Autodesk Inventor part; units mm, degrees
ref_plane "YZ Plane" through (0, 0, 0) normal (1, 0, 0) x (0, 1, 0)
ref_plane "XZ Plane" through (0, 0, 0) normal (0, 1, 0) x (-1, 0, 0)
ref_plane "XY Plane" through (0, 0, 0) normal (0, 0, 1) x (1, 0, 0)
ref_plane "Work Plane1" through (-1.5, 0, 1210) normal (-1, 0, 0) x (0, 0, 1)
sketch "Sketch1" plane through (-1.5, 0, 1210) normal (-1, 0, 0) x (0, 0, 1)
  circle A0 centre (-606.5, 339) radius 1.5
  circle A1 centre (-848.5, 64) radius 1.5
  circle A2 centre (-1090.5, 339) radius 1.5
  circle A3 centre (-848.5, 614) radius 1.5
  circle A4 centre (-364.5, 614) radius 1.5
  circle A5 centre (-364.5, 64) radius 1.5
  circle A6 centre (-122.5, 339) radius 1.5
  circle A7 centre (-122.5, 614) radius 1.5
  circle A8 centre (-122.5, 64) radius 1.5
  circle A9 centre (-364.5, 339) radius 1.5
  circle A10 centre (-606.5, 614) radius 1.5
  circle A11 centre (-1090.5, 614) radius 1.5
  circle A12 centre (-1090.5, 64) radius 1.5
  circle A13 centre (-848.5, 339) radius 1.5
  circle A14 centre (-606.5, 64) radius 1.5
  line L0 (-1211.5, 0) -> (0, 0)
  line L1 (0, 0) -> (0, 1000)
  line L2 (-1211.5, 1000) -> (0, 1000)
  line L3 (-1211.5, 0) -> (-1211.5, 1000)
  line L4 (-25, 76.5) -> (-1186.5, 76.5)
  line L5 (-1186.5, 76.5) -> (-1186.5, 51.5)
  line L6 (-1186.5, 51.5) -> (-25, 51.5)
  line L7 (-25, 51.5) -> (-25, 76.5)
  line L8 (-122.5, 64) -> (-114.6022, 64)
  point P0 (-1210, 0)
  dimension "d0" = 25
  dimension "d1" = 25
  dimension "d2" = 25
ref_plane "Work Plane2" through (-1211.5, 0, -1.5) normal (1, 0, 0) x (0, 0, -1)
sketch "Sketch2" plane through (-1211.5, 0, -1.5) normal (1, 0, 0) x (0, 0, -1)
  line L0 (-25, 51.5) -> (-1186.5, 51.5)
  line L1 (-25, 76.5) -> (-25, 51.5)
  line L2 (-1186.5, 76.5) -> (-25, 76.5)
  line L3 (-1186.5, 51.5) -> (-1186.5, 76.5)
  circle A0 centre (-121, 64) radius 1.5
  circle A1 centre (-363, 64) radius 1.5
  circle A2 centre (-605, 64) radius 1.5
  circle A3 centre (-847, 64) radius 1.5
  circle A4 centre (-1089, 64) radius 1.5
  point P0 (-1.5, 0)
extrude "Extrusion1" add sketch "Sketch2" along normal blind 25
extrude "Extrusion2" add sketch "Sketch1" along normal blind 25 contours L7 L6 L5 L4
ref_plane "Work Plane3" through (-1.5, 0, 1210) normal (-1, 0, 0) x (0, 0, 1)
sketch "Sketch3" plane through (-1.5, 0, 1210) normal (-1, 0, 0) x (0, 0, 1)
  line L0 (-1186.5, 76.5) -> (-1186.5, 51.5)
  line L1 (-1186.5, 51.5) -> (-1210, 51.5)
  line L2 (-1210, 51.5) -> (-1210, 76.5)
  line L3 (-1210, 76.5) -> (-1186.5, 76.5)
  line L4 (-1186.5, 76.5) -> (-1186.5, 51.5)
  line L5 (-1.5, 0) -> (-1.5, 1000)
  line L6 (-25, 76.5) -> (-25, 51.5)
  line L7 (-25, 51.5) -> (-1.5, 51.5)
  line L8 (-1.5, 51.5) -> (-1.5, 76.5)
  line L9 (-1.5, 76.5) -> (-25, 76.5)
  line L10 (-25, 76.5) -> (-25, 51.5)
  point P0 (-1210, 0)
extrude "Extrusion3" add sketch "Sketch3" along normal up to surface (1210 mm away)
sketch "Sketch4" plane through (-1.5, 51.5, 1208.5) normal (0, 0, 1) x (1, 0, 0)
  circle A0 centre (-121, 12.5) radius 1.5
  circle A1 centre (-363, 12.5) radius 1.5
  circle A2 centre (-605, 12.5) radius 1.5
  circle A3 centre (-847, 12.5) radius 1.5
  circle A4 centre (-1089, 12.5) radius 1.5
  point P0 (1.5, -51.5)
hole "Hole1" at (-122.5, 64, 1208.5) at (-606.5, 64, 1208.5) at (-364.5, 64, 1208.5) at (-848.5, 64, 1208.5) at (-1090.5, 64, 1208.5) direction (0, 0, -1) diameter 3 end through all
properties part number "HoneyComb Frame"
For this review, take the finished solid that the model builds, in its own axes (mm). Round coordinates to 2 decimals unless told otherwise and drop trailing zeros. Order: outer loops, then holes, each group sorted by start corner. A loop starts at its lowest first (then second) coordinate and runs counter-clockwise, first axis right, second up. Notation, with made-up numbers: M 64,77.5 L 95,77.5 A23 ccw 95,87.5 Z; hole C 26.25,3.5 d9. An arc over 180 degrees is marked long. Use a Markdown table: item, result. Add a question column.
Item 1: Add section A-A, the plane z = 961.5. Give the boundary of the cut face in (x, y), then the cut area to 3 significant figures.
Item 2: Add section B-B, the plane x = -403.5. Give the boundary of the cut face in (y, z).
Item 3: To check wall thickness, follow line 1 along X through (y, z) = (64, 1195.25); line 2 along Z through (x, y) = (-7.5, 64); line 3 along Y through (x, z) = (-122.5, 1192). State the ranges of each line that lie inside material, in increasing order.
Item 4: Add section C-C, the plane y = 70.5. Give the boundary of the cut face in (x, z).
Geometry results:
| question | item | result |
|---|---|---|
| 1 | outline | M -1211.5,51.5 L -1186.5,51.5 L -1186.5,76.5 L -1211.5,76.5 Z; M -26.5,51.5 L -1.5,51.5 L -1.5,76.5 L -26.5,76.5 Z |
| 1 | area | 1,250 mm² |
| 2 | outline | M 51.5,0 L 76.5,0 L 76.5,23.5 L 51.5,23.5 Z; M 51.5,1185 L 76.5,1185 L 76.5,1208.5 L 51.5,1208.5 Z |
| 3 | line 1 | x = -1211.5 to -1092, -1089 to -850, -847 to -608, -605 to -366, -363 to -124, -121 to -1.5 |
| 3 | line 2 | z = 0 to 118, 121 to 360, 363 to 602, 605 to 844, 847 to 1086, 1089 to 1208.5 |
| 3 | line 3 | y = 51.5 to 62.5, 65.5 to 76.5 |
| 4 | outline | M -1211.5,0 L -1.5,0 L -1.5,1208.5 L -1211.5,1208.5 Z; hole M -1186.5,23.5 L -26.5,23.5 L -26.5,1185 L -1186.5,1185 Z |
